For this review, use the dimensioned drawing (mm, ordinates from the lowest corner) and the shaded views. A direction names the side the tool comes from. Coordinates: 2 decimals unless noted, no trailing zeros. Write each loop counter-clockwise with the first axis right and the second up, starting at its lowest first coordinate (ties: lowest second). Pieces come first, ordered by that corner, then holes. Notation, with made-up numbers: (7.5, 51.5) - (57.5, 51.5) arc R11 ccw to (57.5, 59.5) - close; hole circle Ø1 at (15.5, -32.5). An arc over 180 degrees is marked (long way). One line per item, written item: value.
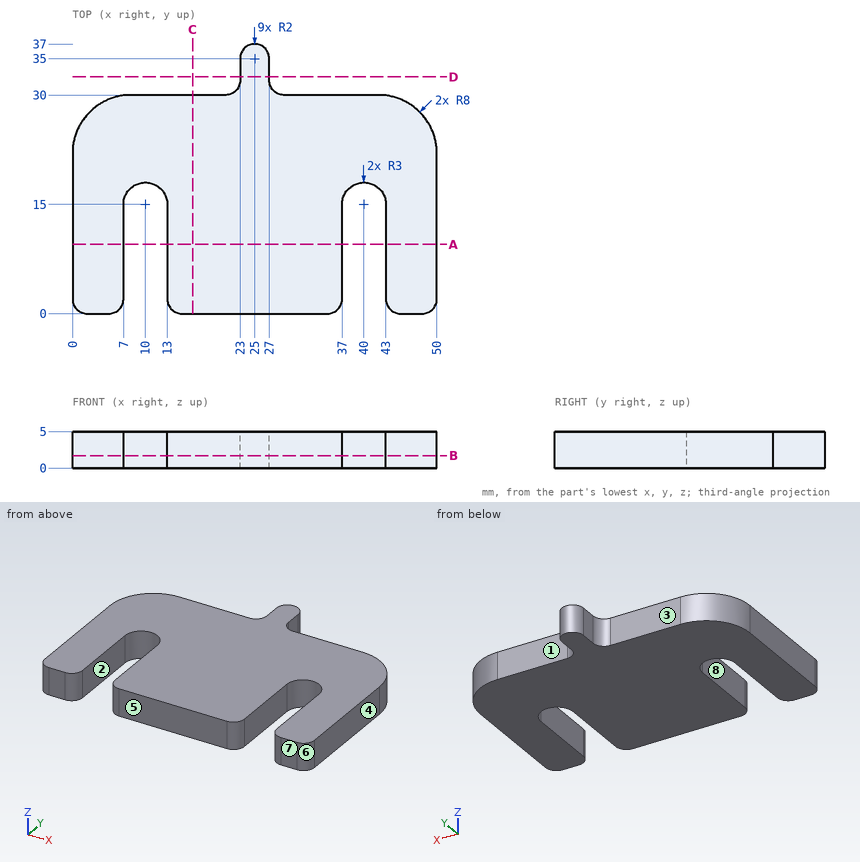
1. Wall thickness on line 1 along X through (y, z) = (12, 0.75); line 2 along Y through (x, z) = (19, 0.65); line 3 along X through (y, z) = (33.5, 2.2): over which ranges is each line inside the solid? List them lowest first.
Answer block:
line 1: x = 0 to 7, 13 to 37, 43 to 50
line 2: y = 0 to 30
line 3: x = 23 to 27
2. Insertion check: pin 1 Ø3 at (x, z) = (12.5, 0.5) entering from -Y; pin 2 Ø2.5 at (y, z) = (33, 3) entering from -X; pin 3 Ø2.5 at (y, z) = (34, 2) entering from +X. Each pin has a flat end and moves straight along its axis. Give the tip position at first contact, or say it passes through.
Answer block:
pin 1: stops at y = 0.27
pin 2: stops at x = 22.98
pin 3: stops at x = 27
3. Consider section C-C, the plane x = 16.5. Write out the cut boundary in (y, z), then the cut area to 3 significant figures.
Answer block:
outline: (0, 0) - (30, 0) - (30, 5) - (0, 5) - close
area: 150 mm^2
4. Mouldability with a two-part tool opening along X and no side actions: class the marked faces 6, 7 and 8 as released by +X, released by -X, zero draft, split by the parting line, or undercut.
Answer block:
face 6: released by +X
face 7: zero draft
face 8: undercut
5. Consider section A-A, the plane y = 9.5. Write out the cut boundary in (x, z).
Answer block:
outline: (0, 0) - (7, 0) - (7, 5) - (0, 5) - close; (13, 0) - (37, 0) - (37, 5) - (13, 5) - close; (43, 0) - (50, 0) - (50, 5) - (43, 5) - close
6. For the marked faces 1, 2, 3, 4 and 5, list the 3-axis set-ups (+Z, -Z, +X, -X, +Y, -Y) from which the entire face can be reached by the end or side of a thin tool; tool diameter is ignored.
Answer block:
face 1: +Z, -Z, +X, +Y
face 2: +Z, -Z, -Y
face 3: +Z, -Z, -X, +Y
face 4: +Z, -Z, +X, +Y, -Y
face 5: +Z, -Z, +X, -X, -Y
7. Consider section D-D, the plane y = 32.5. Write out the cut boundary in (x, z), then the cut area to 3 significant figures.
Answer block:
outline: (23, 0) - (27, 0) - (27, 5) - (23, 5) - close
area: 20.0 mm^2
8. Consider section B-B, the plane z = 1.7. Write out the cut boundary in (x, y), then the cut area to 3 significant figures.
Answer block:
outline: (0, 2) arc R2 ccw to (2, 0) - (5, 0) arc R2 ccw to (7, 2) - (7, 15) arc R3 cw to (13, 15) - (13, 2) arc R2 ccw to (15, 0) - (35, 0) arc R2 ccw to (37, 2) - (37, 15) arc R3 cw to (43, 15) - (43, 2) arc R2 ccw to (45, 0) - (48, 0) arc R2 ccw to (50, 2) - (50, 22) arc R8 ccw to (42, 30) - (29, 30) arc R2 cw to (27, 32) - (27, 35) arc R2 ccw to (23, 35) - (23, 32) arc R2 cw to (21, 30) - (8, 30) arc R8 ccw to (0, 22) - close
area: 1,290 mm^2
